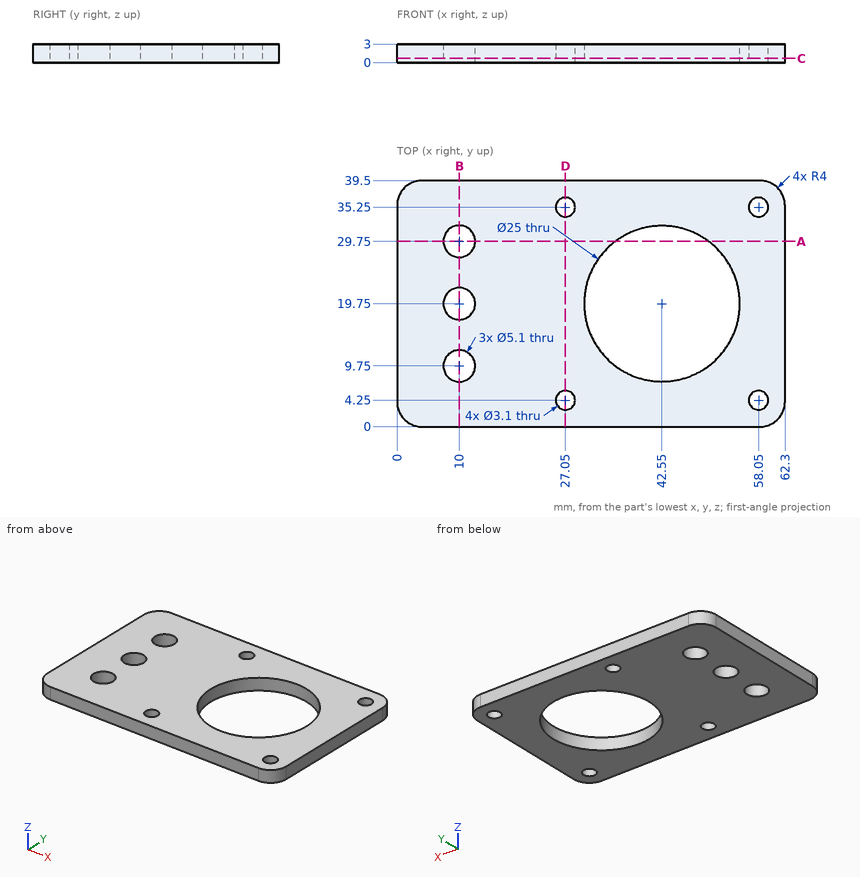
Drawing for the job (mm, zero at the part's lowest x, y, z). Give positions to 0.01 mm unless a question says otherwise; leave off trailing zeros. Loops run counter-clockwise (first coordinate to the right, second up) from the corner with the lowest first, then second, coordinate; pieces in that order, holes last.
1) Band-saw the part on D-D on x = 27.05. List the corners of the cut face in (y, z).
Values follow:
outline: (0, 0) - (2.7, 0) - (2.7, 3) - (0, 3) - close; (5.8, 0) - (33.7, 0) - (33.7, 3) - (5.8, 3) - close; (36.8, 0) - (39.5, 0) - (39.5, 3) - (36.8, 3) - close
2) Probe line 1 along Y through (x, z) = (58.05, 0.7); line 2 along Y through (x, z) = (11, 1.7); line 3 along X through (y, z) = (30.5, 0.9). List the from-to ranges inside material, lowest first.
Values follow:
line 1: y = 0 to 2.7, 5.8 to 33.7, 36.8 to 39.5
line 2: y = 0 to 7.4, 12.1 to 17.4, 22.1 to 27.4, 32.1 to 39.5
line 3: x = 0 to 7.56, 12.44 to 36.17, 48.93 to 62.3
3) Band-saw the part on A-A on y = 29.75. List the corners of the cut face in (x, z).
Values follow:
outline: (0, 0) - (7.45, 0) - (7.45, 3) - (0, 3) - close; (12.55, 0) - (35.05, 0) - (35.05, 3) - (12.55, 3) - close; (50.05, 0) - (62.3, 0) - (62.3, 3) - (50.05, 3) - close
4) Band-saw the part on C-C on z = 0.7. State how many separate pieces and enclosed holes the cut face has, then the cut area to 3 significant figures.
Values follow:
separate pieces: 1
enclosed holes: 8
area: 1,860 mm2
5) Band-saw the part on B-B on x = 10. List the corners of the cut face in (y, z), then the cut area to 3 significant figures.
Values follow:
outline: (0, 0) - (7.2, 0) - (7.2, 3) - (0, 3) - close; (12.3, 0) - (17.2, 0) - (17.2, 3) - (12.3, 3) - close; (22.3, 0) - (27.2, 0) - (27.2, 3) - (22.3, 3) - close; (32.3, 0) - (39.5, 0) - (39.5, 3) - (32.3, 3) - close
area: 72.6 mm2
